Job drawing, mm, ordinate dimensions from the low corner. One solid piece. A direction names the side the tool comes from. Coordinates: 2 decimals unless noted, no trailing zeros. Loops run counter-clockwise (first coordinate to the right, second up) from the corner with the lowest first, then second, coordinate; pieces in that order, holes last. Notation, with made-up numbers: (38.5, 89.5) - (89.5, 89.5) arc R26 cw to (89.5, 122.5) - close; hole circle Ø8 at (-22.5, 16). An arc over 180 degrees is marked (long way). One line per question, with ' | ' between items. Start each with the question number.
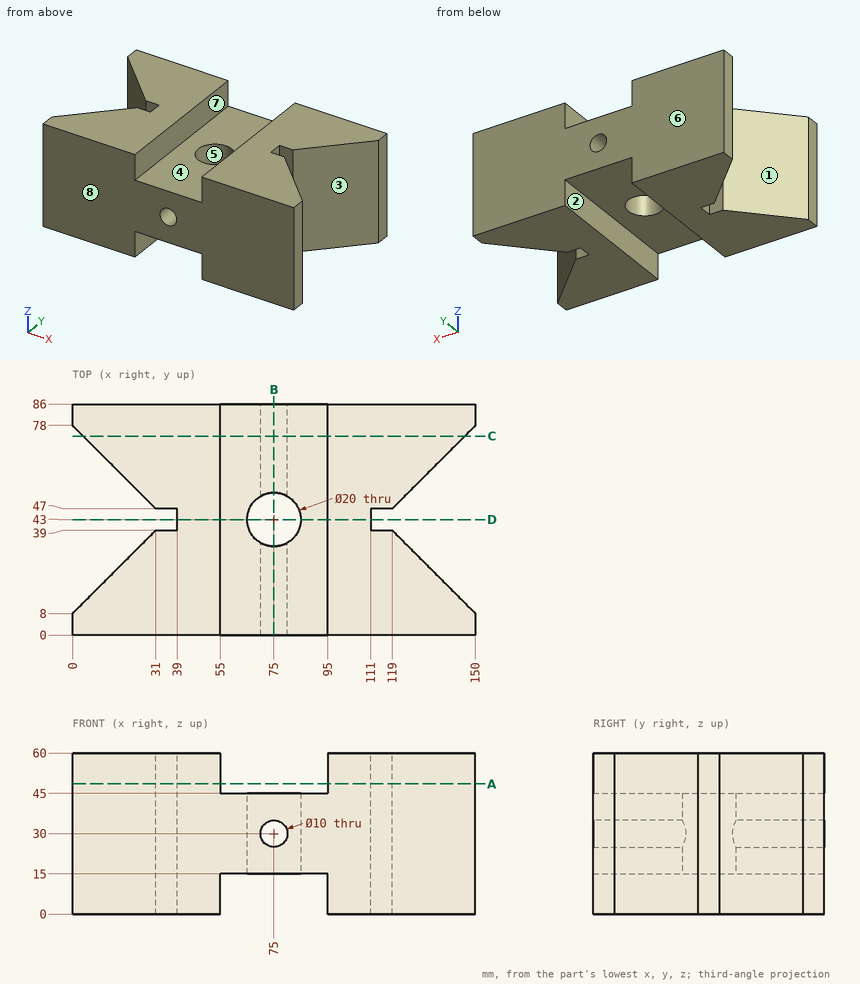
1) Tool access for the marked faces 1, 2, 3 and 4: list every direction of +Z, -Z, +X, -X, +Y, -Y with a clear straight run to the whole face (end or side of a thin tool).
2) Band-saw the part on D-D on y = 43. List the corners of the cut face in (x, z), then the cut area to 3 significant figures.
3) Band-saw the part on C-C on y = 74. List the corners of the cut face in (x, z), then the cut area to 3 significant figures.
4) Mould opens along Y. For the marked faces 5, 6, 7 and 8 say: +Y half, -Y half, draft (parallel to the pull), parting line (faces both ways), or undercut.
5) Band-saw the part on A-A on z = 48.5. List the corners of the cut face in (x, y).
6) Pin check, flat tips, straight feed: pin 1 Ø12 at (y, z) = (56.5, 9) entering from -X; pin 2 Ø4 at (y, z) = (44.5, 25.5) entering from -X; pin 3 Ø12 at (y, z) = (58.5, 9.5) entering from +X. Stop position of each tip, or through.
7) Band-saw the part on B-B on x = 75. List the corners of the cut face in (y, z).
8) Wall check: line 1 along Z through (x, y) = (75, 27.5); line 2 along Z through (x, y) = (64, 32); line 3 along X through (y, z) = (75, 30). Give the ranges that are in metal, low to high. Write a range as [from, to].
Values found:
1) face 1: +Z, -Z, -X | face 2: -Z, +Y, -Y | face 3: +Z, -Z, +X | face 4: +Z, +Y, -Y
2) outline: (39, 0) - (55, 0) - (55, 15) - (65, 15) - (65, 45) - (55, 45) - (55, 60) - (39, 60) - close; (85, 15) - (95, 15) - (95, 0) - (111, 0) - (111, 60) - (95, 60) - (95, 45) - (85, 45) - close | area: 2,520 mm²
3) outline: (4, 0) - (55, 0) - (55, 15) - (95, 15) - (95, 0) - (146, 0) - (146, 60) - (95, 60) - (95, 45) - (55, 45) - (55, 60) - (4, 60) - close; hole circle Ø10 at (75, 30) | area: 7,240 mm²
4) face 5: undercut | face 6: +Y half | face 7: draft | face 8: -Y half
5) outline: (0, 0) - (55, 0) - (55, 86) - (0, 86) - (0, 78) - (31, 47) - (39, 47) - (39, 39) - (31, 39) - (0, 8) - close; (95, 0) - (150, 0) - (150, 8) - (119, 39) - (111, 39) - (111, 47) - (119, 47) - (150, 78) - (150, 86) - (95, 86) - close
6) pin 1: x = 15.5 | pin 2: x = 39 | pin 3: x = 136.5
7) outline: (0, 15) - (33, 15) - (33, 25) - (0, 25) - close; (0, 35) - (33, 35) - (33, 45) - (0, 45) - close; (53, 15) - (86, 15) - (86, 25) - (53, 25) - close; (53, 35) - (86, 35) - (86, 45) - (53, 45) - close
8) line 1: [15, 25], [35, 45] | line 2: [15, 45] | line 3: [3, 70], [80, 147]
